Model file for the job. Use its own axes, mm. Face numbers are marked on the shaded views. A direction names the side the tool comes from. Coordinates: 2 decimals unless noted, no trailing zeros. Loops run counter-clockwise (first coordinate to the right, second up) from the corner with the lowest first, then second, coordinate; pieces in that order, holes last. Notation, with made-up numbers: (9.5, -10.75) -> (14.5, -10.75) arc R13 cw to (14.5, -5.75) -> close; hole circle Ø6 at (73, 22). An arc over 180 degrees is marked (long way). Use one line per item in the form item = value.
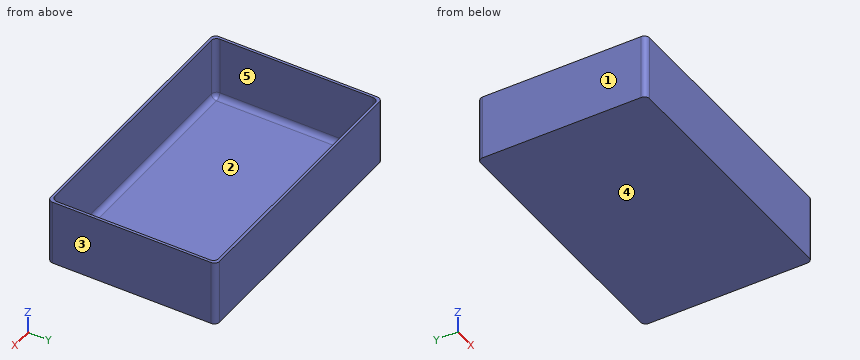
```python
from build123d import *

# Parameters (mm, degrees)
ESQUISSE1_W        = 81.8
ESQUISSE1_H        = 51.4
BOSS_EXTRU_1_DEPTH = 20
COQUE1_T           = -0.8
CONG_1_R           = 1.6


with BuildPart() as part:
    # Esquisse1 → Boss.-Extru.1 (new body)
    with BuildSketch(Plane.XY):
        Rectangle(ESQUISSE1_W, ESQUISSE1_H)
    extrude(amount=BOSS_EXTRU_1_DEPTH)

    # Coque1
    coque1_openings = [part.faces().sort_by_distance(p)[0] for p in [
        (0, 0, 20),
    ]]
    offset(amount=COQUE1_T, openings=coque1_openings, kind=Kind.INTERSECTION)

    # Congé1
    cong_1_edges = [part.edges().sort_by_distance(p)[0] for p in [
        (40.1, 0, 0.8),
        (40.1, -24.9, 10.4),
        (0, 24.9, 0.8),
        (40.1, 24.9, 10.4),
        (-40.1, 0, 0.8),
        (-40.1, 24.9, 10.4),
        (0, -24.9, 0.8),
        (-40.1, -24.9, 10.4),
        (40.9, -25.7, 10),
        (-40.9, -25.7, 10),
        (-40.9, 25.7, 10),
        (40.9, 25.7, 10),
    ]]
    fillet(cong_1_edges, radius=CONG_1_R)


solid = part.part
```
Q1. Mould opens along X. For the marked faces 1, 2 and 3 say: released by +X, released by -X, zero draft, split by the parting line, or undercut.
Result:
face_1 = released by -X
face_2 = undercut
face_3 = released by +X
Q2. Band-saw the part on C-C, the plane z = 10.75. Write the cut outline in (x, y).
Result:
outline = (-40.9, -24.1) arc R1.6 ccw to (-39.3, -25.7) -> (39.3, -25.7) arc R1.6 ccw to (40.9, -24.1) -> (40.9, 24.1) arc R1.6 ccw to (39.3, 25.7) -> (-39.3, 25.7) arc R1.6 ccw to (-40.9, 24.1) -> close; hole (-40.1, -23.3) arc R1.6 ccw to (-38.5, -24.9) -> (38.5, -24.9) arc R1.6 ccw to (40.1, -23.3) -> (40.1, 23.3) arc R1.6 ccw to (38.5, 24.9) -> (-38.5, 24.9) arc R1.6 ccw to (-40.1, 23.3) -> close
Q3. Pin check, flat tip, straight feed: pin 1 Ø23.5 at (x, y) = (-11, -9.5) entering from +Z. Stop position of the tip, or through.
Result:
pin_1 = 0.8
Q4. Band-saw the part on B-B, the plane x = -30.5. Write the cut outline in (y, z).
Result:
outline = (-25.7, 0) -> (25.7, 0) -> (25.7, 20) -> (24.9, 20) -> (24.9, 2.4) arc R1.6 cw to (23.3, 0.8) -> (-23.3, 0.8) arc R1.6 cw to (-24.9, 2.4) -> (-24.9, 20) -> (-25.7, 20) -> close
Q5. Which spindle directions (+Z, -Z, +X, -X, +Y, -Y) get a long thin tool onto all of the face, cutting with end or side? Do the marked faces 4 and 5. Say none if no direction does.
Result:
face_4 = -Z, +X, -X, +Y, -Y
face_5 = +Z
Q6. Wall check: line 1 along X through (y, z) = (17, 6.75); line 2 along Y through (x, z) = (26.5, 6); line 3 along Z through (x, y) = (8.5, 10.5). Give the ranges that are in metal, low to high.
Result:
line_1 = -40.9 to -40.1, 40.1 to 40.9
line_2 = -25.7 to -24.9, 24.9 to 25.7
line_3 = 0 to 0.8
Q7. Band-saw the part on A-A, the plane y = -20. Write the cut outline in (x, z).
Result:
outline = (-40.9, 0) -> (40.9, 0) -> (40.9, 20) -> (40.1, 20) -> (40.1, 2.4) arc R1.6 cw to (38.5, 0.8) -> (-38.5, 0.8) arc R1.6 cw to (-40.1, 2.4) -> (-40.1, 20) -> (-40.9, 20) -> close
